Verification items for the finished model (mm, model axes). Round coordinates to 2 decimals unless told otherwise and drop trailing zeros. Write each loop counter-clockwise with the first axis right and the second up, starting at its lowest first coordinate (ties: lowest second). Pieces come first, ordered by that corner, then holes. Notation, with made-up numbers: M -40,49.5 L -20,49.5 A21 ccw -20,65.5 Z; hole C -1.5,52.5 d4. An arc over 180 degrees is marked long. Use a Markdown table: item, result. Add a question column.
from build123d import *

# Parameters (mm, degrees)
F0_R           = 39.0830403339
F1_DEPTH       = 76.2
F2_R           = 5
F4_D           = 20
F4_DEPTH       = 50
F4_CBORE_D     = 20
F4_CBORE_DEPTH = 30
F4_TIP         = 6.0086061903


with BuildPart() as f1:
    # F0 (on Top) → F1 (new body)
    with BuildSketch(Plane.XY):
        with Locations((-14.6049745381, 0)):
            Circle(F0_R)
    extrude(amount=F1_DEPTH)

    # F2
    f2_edges = [f1.edges().sort_by_distance(p)[0] for p in [
        (24.478066, 0, 38.1),
        (-53.688015, 0, 0),
        (-53.688015, 0, 76.2),
    ]]
    fillet(f2_edges, radius=F2_R)

    # F4
    with Locations(Plane.XY.offset(76.2)):
        with Locations((-14.6049745381, 0)):
            CounterBoreHole(F4_D / 2, F4_CBORE_D / 2, F4_CBORE_DEPTH, depth=F4_DEPTH)
            with Locations((0, 0, -(F4_DEPTH + F4_TIP / 2))):  # 118° drill point
                Cone(0, F4_D / 2, F4_TIP, mode=Mode.SUBTRACT)


solid = f1.part
1. Release check for a two-part mould opening along Y. For faces 1 (the conical face through (-13.001, -0.665, 21.235)), 2 (the flat face through (-15, 0, 0)), 3 (the cylindrical face through (-23.077, -38.154, 37.637)), 4 (the cylindrical face through (-6.669, -6.085, 50.85)) record: +Y half, -Y half, draft (parallel to the pull), parting line (faces both ways), or undercut.
2. Scan lines: line 1 along X through (y, z) = (8.5, 38.5); line 2 along X through (y, z) = (-4.5, 53); line 3 along Y through (x, z) = (-9, 71.5). Record each from-to range of solid material in increasing order. Write a range as from..to.
3. Cross-section at B-B on z = 10. Enter the section's corners in (x, y), plus the area to 3 significant figures.
4. Depth check by flat-ended pin: pin 1 Ø10 at (y, z) = (-24.5, 47.5) entering from -X; pin 2 Ø6 at (y, z) = (20, 58.5) entering from -X; pin 3 Ø6 at (x, z) = (-31, 54) entering from -Y. Enter the tip coordinate at first touch or a pass-through.
5. Cross-section at A-A on z = 29.5. Enter the section's corners in (x, y).
Answer:
| question | item | result |
|---|---|---|
| 1 | face 1 | undercut |
| 1 | face 2 | draft |
| 1 | face 3 | parting line |
| 1 | face 4 | undercut |
| 2 | line 1 | x = -52.75..-19.87, -9.34..23.54 |
| 2 | line 2 | x = -53.43..-23.54, -5.67..24.22 |
| 2 | line 3 | y = -38.67..-8.28, 8.28..38.67 |
| 3 | outline | C -14.6,0 d78.17 |
| 3 | area | 4,800 mm^2 |
| 4 | pin 1 | stops at x = -48.48 |
| 4 | pin 2 | stops at x = -49.8 |
| 4 | pin 3 | stops at y = -36.72 |
| 5 | outline | C -14.6,0 d78.17; hole C -14.6,0 d20 |
